Geometry check sheet. Reference: the model listing, model coordinates, mm. Face numbers are marked on the shaded views. A direction names the side the tool comes from. Coordinates: 2 decimals unless noted, no trailing zeros. Loops run counter-clockwise (first coordinate to the right, second up) from the corner with the lowest first, then second, coordinate; pieces in that order, holes last.
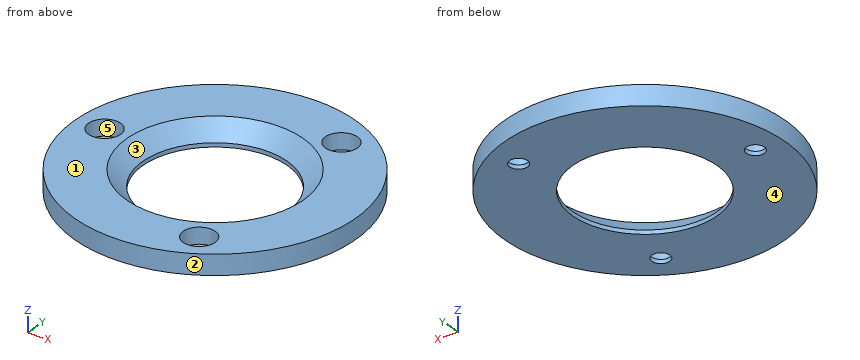
Autodesk Fusion 360 part; units mm, degrees
sketch "Sketch1" plane through (0, 0, 0) normal (0, 0, 1) x (1, 0, 0)
  circle A0 centre (0, 0) radius 18
  circle A1 centre (0, 0) radius 35
  dimension "d1" = 36
  dimension "d2" = 70
extrude "Extrude1" add sketch "Sketch1" along normal blind 5
sketch "Sketch2" plane through (0, 0, 5) normal (0, 0, 1) x (-1, 0, 0)
  circle A0 centre (0, 0) radius 18
  circle A1 centre (0, 0) radius 35
  line L0 (0, 0) -> (28, 0) construction
  line L1 (0, 0) -> (-14, -24.2487) construction
  line L2 (0, 0) -> (-14, 24.2487) construction
  dimension "d5" = 28
  dimension "d8" = 28
  dimension "d13" = 120
  dimension "d14" = 28
  dimension "d15" = 120
hole "Hole1" at (-28, 0, 5) at (14, -24.2487, 5) at (14, 24.2487, 5) direction (0, 0, -1) diameter 4.5 end through all counterbore diameter 8 counterbore depth 4
chamfer "Chamfer1" distance 4 angle 45 1 edges at (-16.7819, 6.5091, 5)
equation "d8 = d5"
equation "d14 = d5"
equation "d15 = d13"
(1) Sectioned sample at C-C on y = 24.5. Record the cut outline in (x, z) (3 decimals).
Findings:
outline: (-24.995, 0) - (11.764, 0) - (11.764, 1) - (10.008, 1) - (10.008, 5) - (-24.995, 5) - close; (16.236, 0) - (24.995, 0) - (24.995, 5) - (17.992, 5) - (17.992, 1) - (16.236, 1) - close
(2) Sectioned sample at D-D on x = -28. Record the cut outline in (y, z), and give its area (4 significant figures).
Findings:
outline: (-21, 0) - (-2.25, 0) - (-2.25, 1) - (-4, 1) - (-4, 5) - (-21, 5) - close; (2.25, 0) - (21, 0) - (21, 5) - (4, 5) - (4, 1) - (2.25, 1) - close
area: 173.5 mm2
(3) Sectioned sample at A-A on x = 0. Record the cut outline in (y, z), and give its area (3 significant figures).
Findings:
outline: (-35, 0) - (-18, 0) - (-18, 1) - (-22, 5) - (-35, 5) - close; (18, 0) - (35, 0) - (35, 5) - (22, 5) - (18, 1) - close
area: 154 mm2
(4) Sectioned sample at B-B on z = 4.15. Record the cut outline in (x, y), and give its area (3 significant figures).
Findings:
outline: circle Ø70 at (0, 0); hole circle Ø8 at (-28, 0); hole circle Ø42.3 at (0, 0); hole circle Ø8 at (14, -24.25); hole circle Ø8 at (14, 24.25)
area: 2,290 mm2
(5) Access from +Z, -Z, +X, -X, +Y, -Y to the whole of each face (thin tool, end or side, straight path). Record for the marked faces 4 and 5.
Findings:
face 4: -Z, +X, -X, +Y, -Y
face 5: +Z
(6) Gauge pin test, flat ends, axial feed: pin 1 Ø2.5 at (x, y) = (-28, 0) entering from -Z; pin 2 Ø1.5 at (x, z) = (-3.5, 2) entering from -Y; pin 3 Ø10 at (x, y) = (15, -2.5) entering from +Z; pin 4 Ø4 at (x, y) = (-18, -3.5) entering from +Z. Record the tip position at first contact, or that the pin passes through.
Findings:
pin 1: passes through
pin 2: stops at y = -34.89
pin 3: stops at z = 3.21
pin 4: stops at z = 3.34
(7) Draft check along Y on the marked faces 1, 2 and 3. Enter one of: +Y half, -Y half, draft (parallel to the pull), parting line (faces both ways), or undercut.
Findings:
face 1: draft
face 2: parting line
face 3: undercut
(8) Scan lines: L1, parallel to Y at x = 14, z = 1.9; L2, parallel to Y at x = 14, z = 0.25; L3, parallel to Z at x = 11.5, y = 23.5. Record each from-to range of solid material in increasing order.
Findings:
L1: y = -32.08 to -28.25, -20.25 to -12.7, 12.7 to 20.25, 28.25 to 32.08
L2: y = -32.08 to -26.5, -22 to -11.31, 11.31 to 22, 26.5 to 32.08
L3: z = 0 to 1
